Source: CAD feature listing. Evaluate the final solid. Frame: model axes, mm. A direction names the side the tool comes from. Coordinates: 2 decimals unless noted, no trailing zeros. Loops run counter-clockwise (first coordinate to the right, second up) from the corner with the lowest first, then second, coordinate; pieces in that order, holes last. Notation, with made-up numbers: (84, -19) -> (111, -19) arc R22 ccw to (111, -12) -> close; hole circle Ø7 at (-37, 30). An arc over 180 degrees is marked (long way). Answer as a JSON object with one key per item and string values. Group by question number.
from build123d import *

# Parameters (mm, degrees)
SKETCH_1_W          = 56
SKETCH_1_H          = 68
EXTRUDE_1_DEPTH     = 0.5
SKETCH_2_R          = 2.5
EXTRUDE_2_DEPTH     = 15
SKETCH_3_W          = 6
SKETCH_3_H          = 10
EXTRUDE_3_DEPTH     = 10
SKETCH_4_R          = 1.6
CUT_EXTRUDE_1_DEPTH = 10
SKETCH_5_R          = 1.6
CUT_EXTRUDE_2_DEPTH = 10
SKETCH_6_R          = 1.6
CUT_EXTRUDE_3_DEPTH = 10
SKETCH_7_R          = 1.6
CUT_EXTRUDE_4_DEPTH = 10


with BuildPart() as part:
    # ｽｹｯﾁ1 → ﾎﾞｽ - 押し出し1 (new, symmetric)
    with BuildSketch(Plane.XY):
        with Locations((5, 6)):
            Rectangle(SKETCH_1_W, SKETCH_1_H)
    extrude(amount=EXTRUDE_1_DEPTH, both=True)

    # ｽｹｯﾁ2 → ﾎﾞｽ - 押し出し2 (add)
    with BuildSketch(Plane.XY.offset(0.5)):
        with Locations((-16, 7)):
            Circle(SKETCH_2_R)
    extrude(amount=EXTRUDE_2_DEPTH)

    # ｽｹｯﾁ3 → ﾎﾞｽ - 押し出し3 (add)
    with BuildSketch(Plane(origin=(0, 0, -0.5), x_dir=(-1, 0, 0), z_dir=(0, 0, -1))):
        with Locations((18, 7)):
            Rectangle(SKETCH_3_W, SKETCH_3_H)
    extrude(amount=EXTRUDE_3_DEPTH)

    # ｽｹｯﾁ4 → ｶｯﾄ - 押し出し1 (cut)
    with BuildSketch(Plane(origin=(0, 0, -0.5), x_dir=(-1, 0, 0), z_dir=(0, 0, -1))):
        with Locations((16, -4)):
            Circle(SKETCH_4_R)
    extrude(amount=-CUT_EXTRUDE_1_DEPTH, mode=Mode.SUBTRACT)

    # ｽｹｯﾁ5 → ｶｯﾄ - 押し出し2 (cut)
    with BuildSketch(Plane.XY.offset(0.5)):
        with Locations((-16, 18)):
            Circle(SKETCH_5_R)
    extrude(amount=-CUT_EXTRUDE_2_DEPTH, mode=Mode.SUBTRACT)

    # ｽｹｯﾁ6 → ｶｯﾄ - 押し出し3 (cut)
    with BuildSketch(Plane.XY.offset(0.5)):
        with Locations((23, 27.5)):
            Circle(SKETCH_6_R)
    extrude(amount=-CUT_EXTRUDE_3_DEPTH, mode=Mode.SUBTRACT)

    # ｽｹｯﾁ7 → ｶｯﾄ - 押し出し4 (cut)
    with BuildSketch(Plane.XY.offset(0.5)):
        with Locations((22, -21)):
            Circle(SKETCH_7_R)
    extrude(amount=-CUT_EXTRUDE_4_DEPTH, mode=Mode.SUBTRACT)


solid = part.part
1. Ray query, L1, parallel to Y at x = -16, z = -0.05; L2, parallel to Y at x = 23, z = -0.1; L3, parallel to Z at x = 1, y = 33.5. Return the intervals inside material, ascending.
2. Section query B-B on y = 7. Return loops of the section in (x, z).
3. Pin query (flat end, axial travel): pin 1 Ø3.5 at (x, y) = (23, 27.5) entering from +Z; pin 2 Ø8 at (y, z) = (7.5, -6.5) entering from +X; pin 3 Ø8 at (y, z) = (5.5, -6) entering from -X. Return the tip coordinate at first contact, or that it passes through.
4. Reachability of faces 5 (the face through (-18, 5.5, 7.9)), 6 (the face through (-21, 7, -5)), 7 (the face through (-18, 2, -5)), 8 (the face through (-18, 7, -10.5)) from +Z, -Z, +X, -X, +Y, -Y: full face, straight path, thin tool, end or side. Return the list, or none.
5. Section query D-D on x = -5.5. Return loops of the section in (y, z).
6. Section query C-C on z = 14. Return loops of the section in (x, y).
7. Section query A-A on y = -21. Return loops of the section in (x, z), then the cut area to 3 significant figures.
8. Mould query, pull axis Y, two halves, no side actions, for faces 1 (the face through (22.792, 29.086, 0.007)), 2 (the face through (-15, 7, -5)), 3 (the face through (21.792, -19.414, 0.007)), 4 (the face through (-18, 12, -5)). Classes: pulls with the +Y half, pulls with the -Y half, needs draft (parallel to the pull), parting line crosses it, or undercut.
Solved:
{
 "1": {"L1": "-28 to -5.6, -2.4 to 16.4, 19.6 to 40", "L2": "-28 to -22.25, -19.75 to 25.9, 29.1 to 40", "L3": "-0.5 to 0.5"},
 "2": {"outline": "(-23, -0.5) -> (-21, -0.5) -> (-21, -10.5) -> (-15, -10.5) -> (-15, -0.5) -> (33, -0.5) -> (33, 0.5) -> (-13.5, 0.5) -> (-13.5, 15.5) -> (-18.5, 15.5) -> (-18.5, 0.5) -> (-23, 0.5) -> close"},
 "3": {"pin 1": "z = 0.5", "pin 2": "x = -15", "pin 3": "x = -21"},
 "4": {"face 5": "+Z", "face 6": "-Z, -X, +Y, -Y", "face 7": "-Z, +X, -X, -Y", "face 8": "-Z, +X, -X, +Y, -Y"},
 "5": {"outline": "(-28, -0.5) -> (40, -0.5) -> (40, 0.5) -> (-28, 0.5) -> close"},
 "6": {"outline": "circle Ø5 at (-16, 7)"},
 "7": {"outline": "(-23, -0.5) -> (20.4, -0.5) -> (20.4, 0.5) -> (-23, 0.5) -> close; (23.6, -0.5) -> (33, -0.5) -> (33, 0.5) -> (23.6, 0.5) -> close", "area": "52.8 mm^2"},
 "8": {"face 1": "undercut", "face 2": "needs draft", "face 3": "undercut", "face 4": "pulls with the +Y half"}
}
